Read the model definition and answer for the solid it produces. Units are mm, in the model's axes. A direction names the side the tool comes from. Round coordinates to 2 decimals unless told otherwise and drop trailing zeros. Order: outer loops, then holes, each group sorted by start corner. A loop starts at its lowest first (then second) coordinate and runs counter-clockwise, first axis right, second up. Notation, with made-up numbers: (-23.5, 88.5) -> (11.5, 88.5) arc R22 ccw to (11.5, 120.5) -> close; hole circle Ø2 at (-11, 37.5). An arc over 180 degrees is marked (long way). One line per item, written item: value. Start each with the question number.
1. The mould has two halves that part along Y. Classify faces 5 (the face through (0, -7.747, 3)), 6 (the face through (-7.62, -5, 3)), 7 (the face through (-1.89, -1.45, 2.5)): released by +Y, released by -Y, zero draft, split by the parting line, or undercut.
2. For faces 1 (the face through (-3.76, -4.77, 2.25)), 2 (the face through (0, 0, 5.08)), 3 (the face through (0, -3, 0)), 4 (the face through (0, -5, 5.08)), determine the directions among +Z, -Z, +X, -X, +Y, -Y from which every point of the face is accessible in a straight line to the end or side of a thin tool.
3. Section B-B (x = -5.08) is taken. Give the vertices of the cut face in (y, z), then the cut area to 3 significant figures.
4. Consider line 1 (X direction, y = -5.05, z = 2.54); line 2 (Y direction, x = 0, z = 3.5); line 3 (X direction, y = -5, z = 1.5). Determine where each line is inside the solid, lowest interval first.
5. Section A-A (z = 2.54) is taken. Give the vertices of the cut face in (x, y).
6. Section C-C (z = 4.5) is taken. Give the vertices of the cut face in (x, y), then the cut area to 3 significant figures.
7. Section D-D (y = -4.5) is taken. Give the vertices of the cut face in (x, z).
8. Flat-ended cylindrical pins translate along their axes: pin 1 Ø3.5 at (x, z) = (-6, 2.5) entering from +Y; pin 2 Ø4.5 at (x, y) = (0, 0) entering from -Z; pin 3 Ø2 at (x, z) = (5.08, 2.54) entering from +Y; pin 4 Ø3.5 at (x, z) = (-5.08, 2.54) entering from +Y. Find the tip coordinate at first contact, or state that the pin passes through.
from build123d import *

# Parameters (mm, degrees)
SKETCH1_R                          = 2.38125
BOSS_EXTRUDE1_DEPTH                = 5.08
SKETCH2_R                          = 3.90525
BOSS_EXTRUDE2_DEPTH                = 1.524
TAP_DRILL_FOR_6_32_TAP1_AT_2_COUNT = 2
TAP_DRILL_FOR_6_32_TAP1_AT_2_PITCH = 10.16
SKETCH6_W                          = 15.24
SKETCH6_H                          = 5.08
SKETCH6_R                          = 1.35255
BOSS_EXTRUDE3_DEPTH                = 3.84175


with BuildPart() as part:
    # Sketch1 → Boss-Extrude1 (new body)
    with BuildSketch(Plane.XY):
        with BuildLine():
            Line((0, -3.90525), (-7.62, -3.90525))
            Line((-7.62, -3.90525), (-7.62, -1.87325))
            Line((-7.62, -1.87325), (-3.426647341, -1.87325))
            ThreePointArc((-3.426647341, -1.87325), (0, 3.90525), (3.426647341, -1.87325))
            Line((3.426647341, -1.87325), (7.62, -1.87325))
            Line((7.62, -1.87325), (7.62, -3.90525))
            Line((7.62, -3.90525), (0, -3.90525))
        make_face()
        Circle(SKETCH1_R, mode=Mode.SUBTRACT)
    extrude(amount=BOSS_EXTRUDE1_DEPTH)

    # Sketch2 → Boss-Extrude2 (add)
    with BuildSketch(Plane.XY.offset(5.08)):
        with Locations(Location((0, 0, 0), (0, 0, 208.664164633))):
            Circle(SKETCH2_R)
    extrude(amount=BOSS_EXTRUDE2_DEPTH)

    # Sketch4 → Tap Drill for #6-32 Tap1 (revolve, cut)
    with BuildSketch(Plane(origin=(-5.08, -1.87325, 2.54), x_dir=(0, 0, 1), z_dir=(1, 0, 0))):
        Polygon((0, 0), (0, 8.43269403), (1.35255, 7.62), (1.35255, 0), align=None)
    tap_drill_for_6_32_tap1 = revolve(axis=Axis((-5.08, 4.47675, 2.54), (0, -1, 0)), mode=Mode.SUBTRACT)

    # Tap Drill for #6-32 Tap1 at 2: Tap Drill for #6-32 Tap1 ×2
    with Locations(*[(i * TAP_DRILL_FOR_6_32_TAP1_AT_2_PITCH, 0, 0) for i in range(1, TAP_DRILL_FOR_6_32_TAP1_AT_2_COUNT)]):
        add(tap_drill_for_6_32_tap1, mode=Mode.SUBTRACT)

    # Sketch6 → Boss-Extrude3 (add)
    with BuildSketch(Plane.XZ.offset(3.90525)):
        with Locations((0, 2.54)):
            Rectangle(SKETCH6_W, SKETCH6_H)
        with Locations(Location((-5.08, 2.54, 0), (0, 0, 90))):
            Circle(SKETCH6_R, mode=Mode.SUBTRACT)
        with Locations(Location((5.08, 2.54, 0), (0, 0, 90))):
            Circle(SKETCH6_R, mode=Mode.SUBTRACT)
    extrude(amount=BOSS_EXTRUDE3_DEPTH)


solid = part.part
Answer:
1. face 5: released by -Y
1. face 6: zero draft
1. face 7: undercut
2. face 1: -Y
2. face 2: -Z
2. face 3: -Z, +X, -X, +Y, -Y
2. face 4: +Z, -Y
3. outline: (-7.75, 0) -> (-1.87, 0) -> (-1.87, 1.19) -> (-7.75, 1.19) -> close; (-7.75, 3.89) -> (-1.87, 3.89) -> (-1.87, 5.08) -> (-7.75, 5.08) -> close
3. area: 13.9 mm^2
4. line 1: -7.62 to -6.43, -3.73 to 3.73, 6.43 to 7.62
4. line 2: -7.75 to -2.38, 2.38 to 3.91
4. line 3: -7.62 to -5.94, -4.22 to 4.22, 5.94 to 7.62
5. outline: (-7.62, -7.75) -> (-6.43, -7.75) -> (-6.43, -1.87) -> (-7.62, -1.87) -> close; (-3.73, -7.75) -> (3.73, -7.75) -> (3.73, -1.87) -> (3.43, -1.87) arc R3.91 ccw (long way) to (-3.43, -1.87) -> (-3.73, -1.87) -> close; (6.43, -7.75) -> (7.62, -7.75) -> (7.62, -1.87) -> (6.43, -1.87) -> close; hole circle Ø4.76 at (0, 0)
6. outline: (-7.62, -7.75) -> (7.62, -7.75) -> (7.62, -1.87) -> (3.43, -1.87) arc R3.91 ccw (long way) to (-3.43, -1.87) -> (-7.62, -1.87) -> close; hole circle Ø4.76 at (0, 0)
6. area: 110 mm^2
7. outline: (-7.62, 0) -> (7.62, 0) -> (7.62, 5.08) -> (-7.62, 5.08) -> close; hole circle Ø2.71 at (-5.08, 2.54); hole circle Ø2.71 at (5.08, 2.54)
8. pin 1: y = -1.87
8. pin 2: z = 5.08
8. pin 3: through
8. pin 4: y = 2.04
